Geometry: final body of the model. Coordinates: model frame, mm. A direction names the side the tool comes from. Round coordinates to 2 decimals unless told otherwise and drop trailing zeros. Write each loop counter-clockwise with the first axis right and the second up, starting at its lowest first coordinate (ties: lowest second). Pieces come first, ordered by that corner, then holes. Notation, with made-up numbers: M -14.5,10.5 L -5.5,10.5 A24 ccw -5.5,34.5 Z; hole C 76.5,75.5 d9. An arc over 180 degrees is marked long. Use one line per item in the form item = value. Start each with the question number.
Item 1: Section query B-B (y = 5). Return loops of the section in (x, z), and give its area (3 significant figures).
Item 2: Ray query, probe 1 along X at (y, z) = (0.65, 0); probe 2 along Z at (x, y) = (15, 0.6); probe 3 along Y at (x, z) = (0, -8.6). Return the intervals inside material, ascending.
Item 3: Section query C-C (z = 0). Return loops of the section in (x, y), and give its area (3 significant figures).
Item 4: Section query D-D (z = 6.25). Return loops of the section in (x, y), and give its area (3 significant figures).
Item 5: Pull-direction query (Z, two-part tool) for faces 4 (the flat face through (0, 12, -9.65)), 5 (the flat face through (-8.1, 22.09, -8.84)), 6 (the flat face through (0, 13, 8.05)); classes: pulls with the +Z half, pulls with the -Z half, needs draft (parallel to the pull), parting line crosses it, or undercut.
Item 6: Reachability of faces 1 (the cylindrical face through (-0.099, 23.635, 8.861)), 2 (the flat face through (13, 6, -9)), 3 (the flat face through (-13, 6, 9)) from +Z, -Z, +X, -X, +Y, -Y: full face, straight path, thin tool, end or side. Return the list, or none.
Item 7: Section query A-A (x = -15). Return loops of the section in (y, z).
Item 8: Pin query (flat end, axial travel): pin 1 Ø3 at (x, y) = (14, 6.5) entering from -Z; pin 2 Ø6 at (x, z) = (4.5, -4.5) entering from +Y; pin 3 Ø1.8 at (y, z) = (6, 9) entering from -X; pin 4 Ø0.5 at (y, z) = (6, -8.5) entering from +X. Return the tip coordinate at first contact, or that it passes through.
Autodesk Inventor part; units mm, degrees
ref_plane "YZ Plane" through (0, 0, 0) normal (1, 0, 0) x (0, 1, 0)
ref_plane "XZ Plane" through (0, 0, 0) normal (0, 1, 0) x (-1, 0, 0)
ref_plane "XY Plane" through (0, 0, 0) normal (0, 0, 1) x (1, 0, 0)
sketch "スケッチ1" plane through (0, 0, 0) normal (0, 1, 0) x (-1, 0, 0)
  line L0 (18.5, 9.65) -> (-18.5, 9.65)
  line L1 (-18.5, 9.65) -> (-18.5, -9.65)
  line L2 (-18.5, -9.65) -> (18.5, -9.65)
  line L3 (18.5, -9.65) -> (18.5, 9.65)
  line L4 (0, 9.65) -> (0, -9.65)
  circle A0 centre (15, 0) radius 2.25
  circle A1 centre (-15, 0) radius 2.25
  point P0 (0, 0)
  point P1 (-15, 0)
  point P2 (0, 0)
  dimension "d0" = 37
  dimension "d1" = 19.3
  dimension "d2" = 30
  dimension "d3" = 4.5
extrude "押し出し1" add sketch "スケッチ1" along normal blind 1.6
sketch "スケッチ2" plane through (-18.5, 0, 9.65) normal (0, 0, 1) x (1, 0, 0)
  line L0 (0, 0) -> (0, 1.6)
  line L1 (5.5, 1.6) -> (5.5, 13.6)
  line L2 (5.5, 13.6) -> (14.0688, 28.4417)
  line L3 (22.9312, 28.4417) -> (31.5, 13.6)
  line L4 (31.5, 13.6) -> (31.5, 1.6)
  line L5 (13.6056, 31) -> (23.0857, 31) construction
  line L6 (0, 0) -> (37, 0)
  arc A0 (22.9312, 28.4417) -> (14.0688, 28.4417) centre (18.5, 25.8833) ccw
  line L7 (37, 0) -> (37, 1.6)
  line L8 (0, 1.6) -> (37, 1.6) construction
  line L9 (31.5, 1.6) -> (37, 1.6) construction
  line L10 (5.5, 1.6) -> (0, 1.6) construction
  line L11 (5.5, 1.6) -> (31.5, 1.6)
  point P0 (18.5, 0)
  point P1 (18.5, 35.8969)
  point P2 (18.5, 0)
  dimension "d6" = 12
  dimension "d7" = 31
  dimension "d14" = 26
  dimension "d15" = 60
extrude "押し出し2" add sketch "スケッチ2" against normal up to surface (19.3 mm away)
sketch "スケッチ3" plane through (18.5, 0, 9.65) normal (1, 0, 0) x (0, 0, -1)
  line L0 (0, 13.6) -> (0, 28.4417)
  line L1 (0, 0) -> (0, 1.6)
  line L2 (0, 0) -> (19.3, 0)
  line L3 (19.3, 0) -> (19.3, 1.6)
  line L4 (19.3, 13.6) -> (19.3, 28.4417)
  line L5 (19.3, 31) -> (19.3, 28.4417)
  line L6 (0, 31) -> (0, 28.4417)
  line L7 (1.6, 31) -> (1.6, 28.6547)
  line L8 (1.6, 28.6547) -> (1.6, 13.6)
  line L9 (1.6, 13.6) -> (1.6, 1.6)
  line L10 (1.6, 1.6) -> (17.7, 1.6)
  line L11 (17.7, 1.6) -> (17.7, 13.6)
  line L12 (17.7, 13.6) -> (17.7, 28.6547)
  line L13 (17.7, 28.6547) -> (17.7, 31)
  line L14 (1.6, 31) -> (17.7, 31)
  line L15 (0, 31) -> (19.3, 31)
  point P0 (9.65, 0)
  dimension "d10" = 1.6
extrude "押し出し3" cut sketch "スケッチ3" against normal through all
fillet "フィレット1" radius 10 4 edges at (13, 13.6, 8.85) (13, 13.6, -8.85) (-13, 13.6, -8.85) (-13, 13.6, 8.85)
sketch "スケッチ4" plane through (18.5, 0, -9.65) normal (0, 0, -1) x (-1, 0, 0)
  arc A0 (22.9312, 28.4417) -> (14.0688, 28.4417) centre (18.5, 25.8833) ccw
  point P0 (18.5, 0)
hole "穴1" at (0, 25.8833, -9.65) direction (0, 0, 1) diameter 4.5 depth 19.3
ref_plane "作業平面1" through (18.5, 0, 0) normal (0, 0, -1) x (-1, 0, 0)
properties part number "mounter" material "アルミニウム 6061"
Working result:
q1.outline = M -13,-9.65 L 13,-9.65 L 13,-8.05 L -13,-8.05 Z; M -13,8.05 L 13,8.05 L 13,9.65 L -13,9.65 Z
q1.area = 83.2 mm²
q2.probe_1 = -18.5 to -17.25, -12.75 to 12.75, 17.25 to 18.5
q2.probe_2 = -9.65 to -2.25, 2.25 to 9.65
q2.probe_3 = 0 to 23.63, 28.13 to 31
q3.outline = M -18.5,0 L -17.25,0 L -17.25,1.6 L -18.5,1.6 Z; M -12.75,0 L 12.75,0 L 12.75,1.6 L -12.75,1.6 Z; M 17.25,0 L 18.5,0 L 18.5,1.6 L 17.25,1.6 Z
q3.area = 44.8 mm²
q4.outline = M -18.5,0 L 18.5,0 L 18.5,1.6 L -18.5,1.6 Z
q4.area = 59.2 mm²
q5.face_4 = pulls with the -Z half
q5.face_5 = needs draft
q5.face_6 = undercut
q6.face_1 = +Z, -Z
q6.face_2 = +Z, -Z, +X, +Y
q6.face_3 = +Z, -Z, -X, +Y
q7.outline = M 0,-9.65 L 1.6,-9.65 L 1.6,-2.25 L 0,-2.25 Z; M 0,2.25 L 1.6,2.25 L 1.6,9.65 L 0,9.65 Z
q8.pin_1 = -9.65
q8.pin_2 = 1.6
q8.pin_3 = -13
q8.pin_4 = 13
